```python
from build123d import *

# Parameters (mm, degrees)
SKETCH1_R           = 6.35
BOSS_EXTRUDE1_DEPTH = 6.35


with BuildPart() as part:
    # Sketch1 → Boss-Extrude1 (new body)
    with BuildSketch(Plane(origin=(0, 0, 0), x_dir=(1, 0, 0), z_dir=(0, 1, 0))):
        with BuildLine():
            Line((-127, 21.997045256), (0, -51.326438931))
            Line((0, -51.326438931), (127, 21.997045256))
            ThreePointArc((127, 21.997045256), (161.697045256, 12.7), (152.4, -21.997045256))
            Line((152.4, -21.997045256), (38.1, -87.988181024))
            Line((38.1, -87.988181024), (38.1, -214.988181024))
            ThreePointArc((38.1, -214.988181024), (0, -253.088181024), (-38.1, -214.988181024))
            Line((-38.1, -214.988181024), (-38.1, -87.988181024))
            Line((-38.1, -87.988181024), (-152.4, -21.997045256))
            ThreePointArc((-152.4, -21.997045256), (-161.697045256, 12.7), (-127, 21.997045256))
        make_face()
        with Locations(Location((-139.7, 0, 0), (0, 0, 270))):
            Circle(SKETCH1_R, mode=Mode.SUBTRACT)
        with Locations(Location((139.7, 0, 0), (0, 0, 270))):
            Circle(SKETCH1_R, mode=Mode.SUBTRACT)
        with BuildLine():
            Line((-9.525, -214.988181024), (-9.525, -95.776438931))
            ThreePointArc((-9.525, -95.776438931), (0, -86.251438931), (9.525, -95.776438931))
            Line((9.525, -95.776438931), (9.525, -214.988181024))
            ThreePointArc((9.525, -214.988181024), (0, -224.513181024), (-9.525, -214.988181024))
        make_face(mode=Mode.SUBTRACT)
    extrude(amount=BOSS_EXTRUDE1_DEPTH)


solid = part.part
```
Model file for the job. Use its own axes, mm. A direction names the side the tool comes from. Give positions to 0.01 mm unless a question says otherwise; leave off trailing zeros. Loops run counter-clockwise (first coordinate to the right, second up) from the corner with the lowest first, then second, coordinate; pieces in that order, holes last. Notation, with made-up numbers: M 88,7.5 L 100,7.5 A7 ccw 100,12.5 Z; hole C 67,77 d8. An arc over 180 degrees is marked long. Use one line per item in the form item = value.
Item 1: Slice it at B-B on z = 0. List the corners of the cut face in (x, y).
Filled in:
outline = M -165.1,0 L -146.05,0 L -146.05,6.35 L -165.1,6.35 Z; M -133.35,0 L -88.9,0 L -88.9,6.35 L -133.35,6.35 Z; M 88.9,0 L 133.35,0 L 133.35,6.35 L 88.9,6.35 Z; M 146.05,0 L 165.1,0 L 165.1,6.35 L 146.05,6.35 Z
Item 2: Drill centre lines: L1, parallel to X at y = 2, z = 0; L2, parallel to X at y = 0.75, z = 196.5 (3 decimals); L3, parallel to X at y = 4.5, z = 1. Where is each one in solid material? Low to high.
Filled in:
L1 = -165.1 to -146.05, -133.35 to -88.9, 88.9 to 133.35, 146.05 to 165.1
L2 = -38.1 to -9.525, 9.525 to 38.1
L3 = -165.08 to -145.97, -133.43 to -87.17, 87.17 to 133.43, 145.97 to 165.08
Item 3: Which spindle directions (+Z, -Z, +X, -X, +Y, -Y) get a long thin tool onto all of the face, cutting with end or side? Do faces 4 (the flat face through (62.61, 3.13, 15.18)), 5 (the cylindrical face through (-0.209, 3.131, 86.254)), 6 (the flat face through (13, 0, 82)). Say none if no direction does.
Filled in:
face_4 = -Z, +Y, -Y
face_5 = +Y, -Y
face_6 = +Z, -Z, +X, -X, -Y
Item 4: Slice it at C-C on x = 139.7. List the corners of the cut face in (y, z), and give its area (3 significant figures).
Filled in:
outline = M 0,-25.4 L 6.35,-25.4 L 6.35,-6.35 L 0,-6.35 Z; M 0,6.35 L 6.35,6.35 L 6.35,29.33 L 0,29.33 Z
area = 267 mm^2
Item 5: Two-plate mould, pull along Z, no slides. Class faces 1 (the flat face through (96.1, 3.1, 54.5)), 2 (the cylindrical face through (0.21, 3.13, 224.51)), 3 (the flat face through (-64.39, 3.13, 14.15)): released by +Z, released by -Z, zero draft, split by the parting line, or undercut.
Filled in:
face_1 = released by +Z
face_2 = undercut
face_3 = released by -Z
Item 6: Slice it at A-A on z = 165.5. List the corners of the cut face in (x, y) (3 decimals).
Filled in:
outline = M -38.1,0 L -9.525,0 L -9.525,6.35 L -38.1,6.35 Z; M 9.525,0 L 38.1,0 L 38.1,6.35 L 9.525,6.35 Z
Item 7: Flat gauge pins, fed straight in: pin 1 Ø3 at (x, y) = (-109, 5) entering from -Z; pin 2 Ø1.9 at (y, z) = (2, 140.5) entering from -X; pin 3 Ø3 at (y, z) = (3, 121.5) entering from +X; pin 4 Ø10 at (x, z) = (-139.7, 0) entering from +Y. Where does each tip first touch, or does it go through?
Filled in:
pin_1 = -12.47
pin_2 = -38.1
pin_3 = 38.1
pin_4 = through
Item 8: Slice it at D-D on y = 2.75. List the corners of the cut face in (x, z) (3 decimals).
Filled in:
outline = M -152.4,21.997 A25.4 ccw -127,-21.997 L 0,51.326 L 127,-21.997 A25.4 ccw 152.4,21.997 L 38.1,87.988 L 38.1,214.988 A38.1 ccw -38.1,214.988 L -38.1,87.988 Z; hole C -139.7,0 d12.7; hole M -9.525,95.776 A9.525 ccw 9.525,95.776 L 9.525,214.988 A9.525 ccw -9.525,214.988 Z; hole C 139.7,0 d12.7
